Source: three-view drawing plus pictorial views. Frame: mm from the lowest corner of the part. Give positions to 0.01 mm unless a question says otherwise; leave off trailing zeros. Order: outer loops, then holes, each group sorted by start corner. A loop starts at its lowest first (then second) coordinate and runs counter-clockwise, first axis right, second up. Notation, with made-up numbers: (26.25, -37.5) - (71.25, -37.5) arc R20 cw to (71.25, -24.5) - close; hole circle Ø1 at (-15.5, 8). An arc over 180 degrees is marked (long way). Answer in a Markdown table with one row per item. Add a question column.
1. Section query C-C on z = 11.5. Return loops of the section in (x, y), and give its area (3 significant figures).
2. Section query D-D on x = 39.5. Return loops of the section in (y, z) (1 decimal).
3. Ray query, line 1 (Y direction, x = 3.5, z = 10.75) (1 decimal); line 2 (X direction, y = 4, z = 5.25) (1 decimal); line 3 (X direction, y = 5, z = 15) (1 decimal). Return the intervals inside material, ascending. Write a range as [from, to].
4. Contact query for flat-ended pins moving along their axis: pin 1 (2 mm diameter, centred on x = 17.5, z = 13.5, fed in from +Y) (1 decimal); pin 2 (2 mm diameter, centred on x = 31, z = 20.5, fed in from -Y) (1 decimal); pin 3 (3 mm diameter, centred on x = 6.5, z = 19.5, fed in from -Y). Output: stop coordinate, or through.
5. Section query A-A on y = 5. Return loops of the section in (x, z) (1 decimal), and give its area (3 significant figures).
6. Section query B-B on x = 5. Return loops of the section in (y, z).
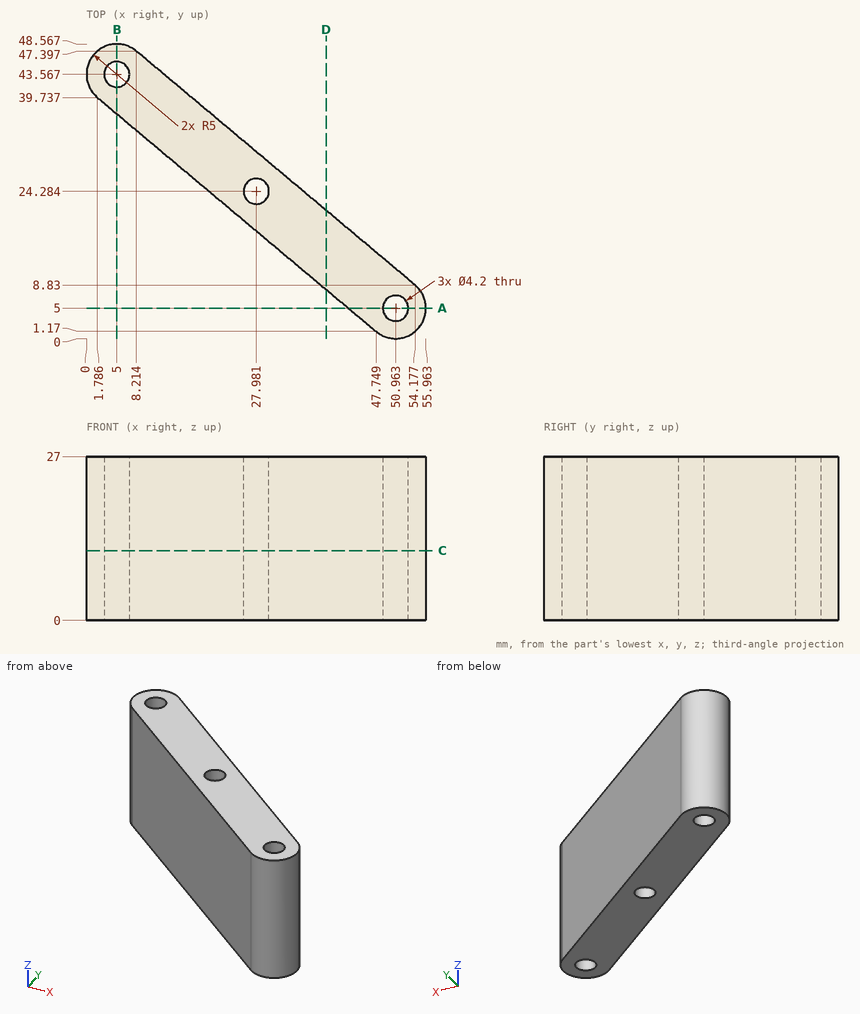
Answer:
| question | item | result |
|---|---|---|
| 1 | outline | (1.79, 39.74) - (47.75, 1.17) arc R5 ccw to (54.18, 8.83) - (8.21, 47.4) arc R5 ccw to start; hole circle Ø4.2 at (5, 43.57); hole circle Ø4.2 at (27.98, 24.28); hole circle Ø4.2 at (50.96, 5) |
| 1 | area | 637 mm² |
| 2 | outline | (8.1, 0) - (21.1, 0) - (21.1, 27) - (8.1, 27) - close |
| 3 | line 1 | y = [38.3, 42.1], [45, 48.3] |
| 3 | line 2 | x = [44.4, 49.1], [52.8, 55.9] |
| 3 | line 3 | x = [43.2, 48.9], [53.1, 56] |
| 4 | pin 1 | stops at y = 40.4 |
| 4 | pin 2 | stops at y = 14.4 |
| 4 | pin 3 | stops at y = 34.52 |
| 5 | outline | (43.2, 0) - (48.9, 0) - (48.9, 27) - (43.2, 27) - close; (53.1, 0) - (56, 0) - (56, 27) - (53.1, 27) - close |
| 5 | area | 232 mm² |
| 6 | outline | (37.04, 0) - (41.47, 0) - (41.47, 27) - (37.04, 27) - close; (45.67, 0) - (48.57, 0) - (48.57, 27) - (45.67, 27) - close |
